from build123d import *

# Parameters (mm, degrees)
SKETCH_1_R      = 15
EXTRUDE_1_DEPTH = 20
SHELL_1_T       = -0.5
FILLET_1_R      = 3


with BuildPart() as part:
    # 草图1 → 凸台-拉伸1 (new body)
    with BuildSketch(Plane.XY):
        Circle(SKETCH_1_R)
    extrude(amount=EXTRUDE_1_DEPTH)

    # 抽壳1
    shell_1_openings = [part.faces().sort_by_distance(p)[0] for p in [
        (0, 0, 0),
    ]]
    offset(amount=SHELL_1_T, openings=shell_1_openings, kind=Kind.INTERSECTION)

    # 圆角1
    fillet_1_edges = [part.edges().sort_by_distance(p)[0] for p in [
        (-15, 0, 20),
    ]]
    fillet(fillet_1_edges, radius=FILLET_1_R)


solid = part.part
The listing builds one solid part. Answer for the finished solid, in the listing's coordinates (mm). Round coordinates to 2 decimals unless told otherwise and drop trailing zeros. Order: outer loops, then holes, each group sorted by start corner. A loop starts at its lowest first (then second) coordinate and runs counter-clockwise, first axis right, second up. Notation, with made-up numbers: M 78,23.25 L 123,23.25 A24 cw 123,61.25 Z; hole C -25.5,0 d11. An arc over 180 degrees is marked long. Answer in a Markdown table with one row per item. Add a question column.
1) Determine the mould class of faces 1 (the face through (6.691, -12.864, 9.614)), 2 (the face through (-14.985, 0.66, 8.381)), 3 (the face through (0, 0, 19.5)), 4 (the face through (0, 0, 20)) for opening direction Y: pulls with the +Y half, pulls with the -Y half, needs draft (parallel to the pull), parting line crosses it, or undercut.
2) The part is cut by section A-A on z = 13. Determine the outline of the cut face in (x, y), plus the area to 3 significant figures.
3) Consider line 1 along Y through (x, z) = (0, 5.25); line 2 along Z through (x, y) = (9, -7.5); line 3 along Y through (x, z) = (10, 5.25). Determine where each line is inside the solid, lowest interval first. Write a range as from..to.
4) Flat-ended cylindrical pins translate along their axes: pin 1 Ø1.5 at (y, z) = (5.5, 17.5) entering from +X; pin 2 Ø10 at (x, y) = (-2.5, -1) entering from -Z; pin 3 Ø6 at (x, z) = (3, 10) entering from -Y; pin 4 Ø5 at (y, z) = (7.5, 5.5) entering from -X. Find the tip coordinate at first contact, or state that the pin passes through.
Findings below:
| question | item | result |
|---|---|---|
| 1 | face 1 | undercut |
| 1 | face 2 | parting line crosses it |
| 1 | face 3 | undercut |
| 1 | face 4 | needs draft |
| 2 | outline | C 0,0 d30; hole C 0,0 d29 |
| 2 | area | 46.3 mm² |
| 3 | line 1 | y = -15..-14.5, 14.5..15 |
| 3 | line 2 | z = 19.5..20 |
| 3 | line 3 | y = -11.18..-10.5, 10.5..11.18 |
| 4 | pin 1 | stops at x = 14.2 |
| 4 | pin 2 | stops at z = 19.5 |
| 4 | pin 3 | stops at y = -15 |
| 4 | pin 4 | stops at x = -14.14 |
